Can you work these out from the drawing? Everything is in mm from the part's minimum corner. A direction names the side the tool comes from. Give positions to 0.01 mm unless a question says otherwise; leave off trailing zeros. Write each loop counter-clockwise with the first axis right and the second up, starting at its lowest first coordinate (ties: lowest second). Pieces come first, ordered by that corner, then holes. Notation, with made-up numbers: (70.25, 69) -> (110.25, 69) arc R14 cw to (110.25, 73) -> close; hole circle Ø5 at (-22, 61.5). An arc over 180 degrees is marked (long way). Write item = value, one per line. Start each with the question number.
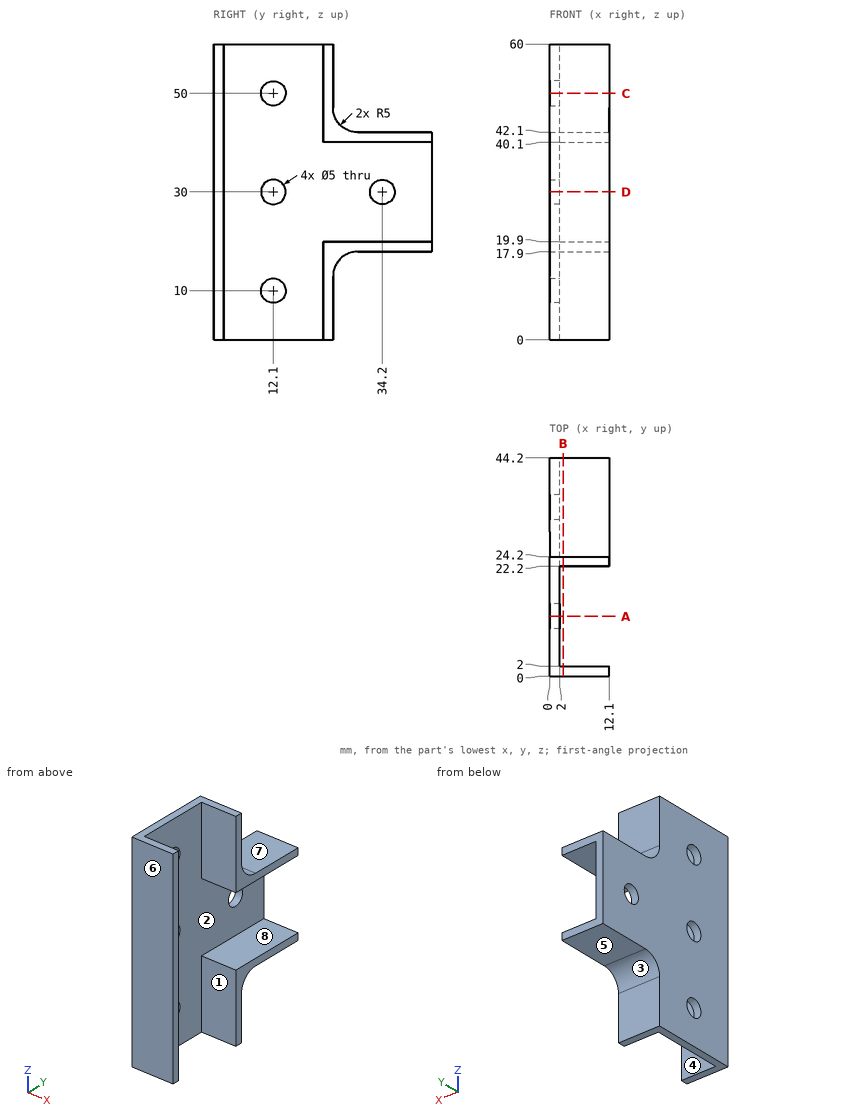
(1) I'm going to push flat-ended pins straight in: pin 1 (3 mm diameter, centred on x = 3, y = 37, fed in from +Z); pin 2 (4 mm diameter, centred on y = 12.1, z = 10, fed in from -X); pin 3 (3 mm diameter, centred on x = 9.5, y = 34, fed in from -Z); pin 4 (1 mm diameter, centred on x = 10.5, y = 26, fed in from +Z). Where does each tip first touch, or does it pass through?
(2) Imagine slicing it at D-D (z = 30). Please give me the cut outline in (x, y), then the cut area to 3 significant figures.
(3) Imagine slicing it at C-C (z = 50). Please give me the cut outline in (x, y), then the cut area to 3 significant figures.
(4) Imagine slicing it at B-B (x = 2.75). Please give me the cut outline in (y, z), then the cut area to 3 significant figures.
(5) On a 3-axis mill with a long thin cutter (end or side, diameter ignored), from which of +Z, -Z, +X, -X, +Y, -Y can I reach the whole of each face in a straight line? I mean the marked faces 4, 5, 6, 7 and 8. Say none if no direction works.
(6) If I drill on line 1 along Y through (x, z) = (0.55, 10); line 2 along Y through (x, z) = (2.5, 13); line 3 along Z through (x, y) = (4.75, 33.5), over which ranges is the centre line in solid material (lowest first)? Write a range as from..to.
(7) We'd pull the mould along Z, two halves only. Please class the marked faces 1, 2 and 3: released by +Z, released by -Z, zero draft, split by the parting line, or undercut.
(8) Imagine slicing it at A-A (y = 12.1). Please give me the cut outline in (x, z).
Answers below:
q1.pin_1 = 42.1
q1.pin_2 = through
q1.pin_3 = 17.9
q1.pin_4 = 43.74
q2.outline = (0, 0) -> (12.1, 0) -> (12.1, 2) -> (2, 2) -> (2, 9.6) -> (0, 9.6) -> close; (0, 14.6) -> (2, 14.6) -> (2, 31.7) -> (0, 31.7) -> close; (0, 36.7) -> (2, 36.7) -> (2, 44.2) -> (0, 44.2) -> close
q2.area = 88.6 mm^2
q3.outline = (0, 0) -> (12.1, 0) -> (12.1, 2) -> (2, 2) -> (2, 9.6) -> (0, 9.6) -> close; (0, 14.6) -> (2, 14.6) -> (2, 22.2) -> (12.1, 22.2) -> (12.1, 24.2) -> (0, 24.2) -> close
q3.area = 78.8 mm^2
q4.outline = (0, 0) -> (2, 0) -> (2, 60) -> (0, 60) -> close; (22.2, 0) -> (24.2, 0) -> (24.2, 12.9) arc R5 cw to (29.2, 17.9) -> (44.2, 17.9) -> (44.2, 19.9) -> (22.2, 19.9) -> close; (22.2, 40.1) -> (44.2, 40.1) -> (44.2, 42.1) -> (29.2, 42.1) arc R5 cw to (24.2, 47.1) -> (24.2, 60) -> (22.2, 60) -> close
q4.area = 290 mm^2
q5.face_4 = +Z, -Z, +X
q5.face_5 = -Z, +X, -X, +Y
q5.face_6 = +Z, -Z, +X, -X, -Y
q5.face_7 = +Z, +X, -X, +Y
q5.face_8 = +X, +Y
q6.line_1 = 0..9.6, 14.6..24.2
q6.line_2 = 0..2, 22.2..24.2
q6.line_3 = 17.9..19.9, 40.1..42.1
q7.face_1 = zero draft
q7.face_2 = undercut
q7.face_3 = released by -Z
q8.outline = (0, 0) -> (2, 0) -> (2, 7.5) -> (0, 7.5) -> close; (0, 12.5) -> (2, 12.5) -> (2, 27.5) -> (0, 27.5) -> close; (0, 32.5) -> (2, 32.5) -> (2, 47.5) -> (0, 47.5) -> close; (0, 52.5) -> (2, 52.5) -> (2, 60) -> (0, 60) -> close
